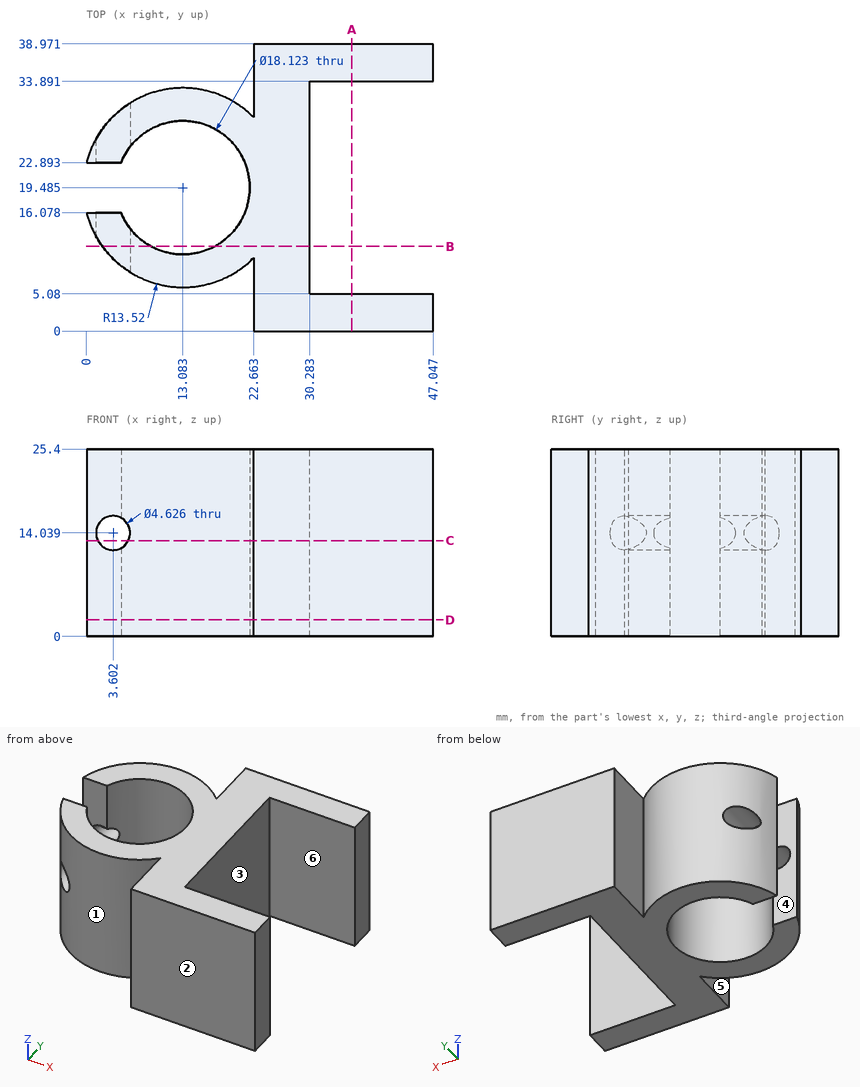
Geometry: see drawing. Coordinates: mm, zero at the bounding-box minimum. A direction names the side the tool comes from. Coordinates: 2 decimals unless noted, no trailing zeros. Order: outer loops, then holes, each group sorted by start corner. A loop starts at its lowest first (then second) coordinate and runs counter-clockwise, first axis right, second up. Notation, with made-up numbers: M -4.75,76 L 0.25,76 A15 ccw 0.25,90 Z; hole C 26,68.25 d8. An arc over 180 degrees is marked long. Write each question's results on one line, items separated by ' | '. Start each with the question number.
1) Contact query for flat-ended pins moving along their axis: pin 1 Ø6 at (y, z) = (35, 14.5) entering from -X (1 decimal); pin 2 Ø6 at (x, z) = (3.6, 14.04) entering from -Y; pin 3 Ø8 at (y, z) = (33.5, 13.5) entering from -X; pin 4 Ø6 at (x, y) = (17.5, 16.5) entering from +Z. Output: stop coordinate, or through.
2) Section query A-A (x = 36). Return the cut outline in (y, z).
3) Line query: line 1 (Y direction, x = 34, z = 7); line 2 (X direction, y = 25.5, z = 19.25) (1 decimal); line 3 (Y direction, x = 16, z = 7) (1 decimal). Output: solid intervals per line, ascending. Write a range as from..to.
4) Section query B-B (y = 11.5). Return the cut outline in (x, z).
5) Draft query along X for the marked faces 1, 2 and 3. Return one class per face: released by +X, released by -X, zero draft, split by the parting line, or undercut.
6) Section query C-C (z = 13). Return the cut outline in (x, y) (1 decimal).
7) Section query D-D (z = 2.25). Return the cut outline in (x, y) (1 decimal).
8) Access query for the marked faces 4, 5 and 6. Directions: +Z, -Z, +X, -X, +Y, -Y. A direction counts if a zero-diameter tool reaches every point of the face in a straight line with its end or side. Return the directions, or none.
Answers:
1) pin 1: stops at x = 8 | pin 2: stops at y = 7.62 | pin 3: stops at x = 4.4 | pin 4: passes through
2) outline: M 0,0 L 5.08,0 L 5.08,25.4 L 0,25.4 Z; M 33.89,0 L 38.97,0 L 38.97,25.4 L 33.89,25.4 Z
3) line 1: y = 0..5.08, 33.89..38.97 | line 2: x = 1..6.3, 19.9..30.3 | line 3: y = 6.3..10.9, 28.1..32.7
4) outline: M 2.17,0 L 8.8,0 L 8.8,25.4 L 2.17,25.4 L 2.17,15.86 A2.31 cw long 2.17,12.22 Z; M 17.37,0 L 30.28,0 L 30.28,25.4 L 17.37,25.4 Z
5) face 1: undercut | face 2: zero draft | face 3: released by +X
6) outline: M 0,16.1 A13.5 ccw 1.5,12.5 L 1.5,16.1 Z; M 0,22.9 L 1.5,22.9 L 1.5,26.5 A13.5 ccw Z; M 5.7,8.2 A13.5 ccw 22.7,9.9 L 22.7,0 L 47,0 L 47,5.1 L 30.3,5.1 L 30.3,33.9 L 47,33.9 L 47,39 L 22.7,39 L 22.7,29 A13.5 ccw 5.7,30.8 L 5.7,24.7 A9.1 cw long 5.7,14.3 Z
7) outline: M 0,16.1 A13.5 ccw 22.7,9.9 L 22.7,0 L 47,0 L 47,5.1 L 30.3,5.1 L 30.3,33.9 L 47,33.9 L 47,39 L 22.7,39 L 22.7,29 A13.5 ccw 0,22.9 L 4.7,22.9 A9.1 cw long 4.7,16.1 Z
8) face 4: +Z, -Z, -X | face 5: +Z, -Z, -Y | face 6: +Z, -Z, +X
